Could you check a few things on this model? Use its own coordinates, in mm. A direction names the side the tool comes from. Give positions to 0.01 mm unless a question says otherwise; leave off trailing zeros. Order: outer loops, then holes, each group sorted by start corner. A loop starts at its lowest first (then second) coordinate and runs counter-clockwise, first axis right, second up.
from build123d import *

# Parameters (mm, degrees)
SKETCH_1_R          = 24
SKETCH_1_R_2        = 1.75
EXTRUDE_1_DEPTH     = 8
FILLET_1_R          = 10
FILLET_3_R          = 10
FILLET_8_R          = 23
FILLET_9_R          = 23
SKETCH_3_R          = 2
CUT_EXTRUDE_1_DEPTH = 196.43671136
RIB_1_REACH         = 197.437
SKETCH_6_WALL_W     = 465.474103638
SKETCH_6_WALL_H     = 8
EXTRUDE_START       = 8
SKETCH_11_W         = 116.312569084
SKETCH_11_H         = 40.000018321
SKETCH_11_R         = 2
EXTRUDE_2_DEPTH     = 8
FILLET_11_R         = 5


with BuildPart() as part:
    # 草图1 → 凸台-拉伸1 (new body)
    with BuildSketch(Plane.XY):
        with BuildLine():
            Line((-100, -20), (100, -20))
            ThreePointArc((100, -20), (189.532340636, 0), (100, 20))
            Line((100, 20), (-100, 20))
            Line((-100, 20), (-100, -20))
        make_face()
        with Locations((142.532340636, 0)):
            Circle(SKETCH_1_R, mode=Mode.SUBTRACT)
        with Locations((123.782340636, 32.475952642)):
            Circle(SKETCH_1_R_2, mode=Mode.SUBTRACT)
        with Locations((107.293867357, 12.825755375)):
            Circle(SKETCH_1_R_2, mode=Mode.SUBTRACT)
        with Locations((107.293867357, -12.825755375)):
            Circle(SKETCH_1_R_2, mode=Mode.SUBTRACT)
        with Locations((123.782340636, -32.475952642)):
            Circle(SKETCH_1_R_2, mode=Mode.SUBTRACT)
        with Locations((149.044147299, -36.930290738)):
            Circle(SKETCH_1_R_2, mode=Mode.SUBTRACT)
        with Locations((171.259007253, -24.104535363)):
            Circle(SKETCH_1_R_2, mode=Mode.SUBTRACT)
        with Locations((180.032340636, 0)):
            Circle(SKETCH_1_R_2, mode=Mode.SUBTRACT)
        with Locations((171.259007253, 24.104535363)):
            Circle(SKETCH_1_R_2, mode=Mode.SUBTRACT)
        with Locations((149.044147299, 36.930290738)):
            Circle(SKETCH_1_R_2, mode=Mode.SUBTRACT)
    extrude(amount=EXTRUDE_1_DEPTH)

    # 圆角1
    fillet_1_edges = [part.edges().sort_by_distance(p)[0] for p in [
        (-100, 20, 4),
    ]]
    fillet(fillet_1_edges, radius=FILLET_1_R)

    # 圆角3
    fillet_3_edges = [part.edges().sort_by_distance(p)[0] for p in [
        (-100, -20, 4),
    ]]
    fillet(fillet_3_edges, radius=FILLET_3_R)

    # 圆角8
    fillet_8_edges = [part.edges().sort_by_distance(p)[0] for p in [
        (100, -20, 4),
    ]]
    fillet(fillet_8_edges, radius=FILLET_8_R)

    # 圆角9
    fillet_9_edges = [part.edges().sort_by_distance(p)[0] for p in [
        (100, 20, 4),
    ]]
    fillet(fillet_9_edges, radius=FILLET_9_R)

    # 草图3 → 切除-拉伸1 (cut, through all)
    with BuildSketch(Plane.XY.offset(8)):
        with Locations((-86.637479545, 10)):
            Circle(SKETCH_3_R)
        with Locations((-86.610408267, -9.999981679)):
            Circle(SKETCH_3_R)
        with Locations((-76.637479545, 10)):
            Circle(SKETCH_3_R)
        with Locations((-76.610408267, -9.999981679)):
            Circle(SKETCH_3_R)
        with Locations((-46.637479545, 10)):
            Circle(SKETCH_3_R)
        with Locations((-46.610408267, -9.999981679)):
            Circle(SKETCH_3_R)
        with Locations((-36.637479545, 10)):
            Circle(SKETCH_3_R)
        with Locations((-36.610408267, -9.999981679)):
            Circle(SKETCH_3_R)
        with Locations((-6.637479545, 10)):
            Circle(SKETCH_3_R)
        with Locations((-6.610408267, -9.999981679)):
            Circle(SKETCH_3_R)
        with Locations((3.362520455, 10)):
            Circle(SKETCH_3_R)
        with Locations((3.389591733, -9.999981679)):
            Circle(SKETCH_3_R)
        with Locations((33.362520455, 10)):
            Circle(SKETCH_3_R)
        with Locations((33.389591733, -9.999981679)):
            Circle(SKETCH_3_R)
        with Locations((43.362520455, 10)):
            Circle(SKETCH_3_R)
        with Locations((43.389591733, -9.999981679)):
            Circle(SKETCH_3_R)
        with Locations((63.247313172, 10)):
            Circle(SKETCH_3_R)
        with Locations((84.747313172, 10)):
            Circle(SKETCH_3_R)
        with Locations((84.747313172, -11.5)):
            Circle(SKETCH_3_R)
        with Locations((63.247313172, -11.5)):
            Circle(SKETCH_3_R)
    extrude(amount=-CUT_EXTRUDE_1_DEPTH, mode=Mode.SUBTRACT)

    # 草图6 wall → 筋1 (add, up to next)
    with BuildSketch(Plane(origin=(69.41709698, 24.435714285, 8), x_dir=(0.992506131536, 0.122194839758, 0), z_dir=(-0.122194839758, 0.992506131536, 0)), mode=Mode.PRIVATE) as rib_1_sk1:
        with Locations((0, 4)):
            Rectangle(SKETCH_6_WALL_W, SKETCH_6_WALL_H)
    rib_1_tool1 = extrude(rib_1_sk1.sketch, amount=-RIB_1_REACH, mode=Mode.PRIVATE) - part.part
    add(rib_1_tool1.solids().sort_by_distance((69.41709698, 24.435714285, 8))[0])

    # 草图11 → 凸台-拉伸2 (add)
    with BuildSketch(Plane.XY.offset(8).offset(EXTRUDE_START)):
        with Locations((-1.623943906, 9.161e-06)):
            Rectangle(SKETCH_11_W, SKETCH_11_H)
        with Locations((-46.637479545, 10)):
            Circle(SKETCH_11_R, mode=Mode.SUBTRACT)
        with Locations((-36.637479545, 10)):
            Circle(SKETCH_11_R, mode=Mode.SUBTRACT)
        with Locations((-36.610408267, -9.999981679)):
            Circle(SKETCH_11_R, mode=Mode.SUBTRACT)
        with Locations((-46.610408267, -9.999981679)):
            Circle(SKETCH_11_R, mode=Mode.SUBTRACT)
        with Locations((-6.637479545, 10)):
            Circle(SKETCH_11_R, mode=Mode.SUBTRACT)
        with Locations((-6.610408267, -9.999981679)):
            Circle(SKETCH_11_R, mode=Mode.SUBTRACT)
        with Locations((3.389591733, -9.999981679)):
            Circle(SKETCH_11_R, mode=Mode.SUBTRACT)
        with Locations((3.362520455, 10)):
            Circle(SKETCH_11_R, mode=Mode.SUBTRACT)
        with Locations((33.362520455, 10)):
            Circle(SKETCH_11_R, mode=Mode.SUBTRACT)
        with Locations((43.362520455, 10)):
            Circle(SKETCH_11_R, mode=Mode.SUBTRACT)
        with Locations((43.389591733, -9.999981679)):
            Circle(SKETCH_11_R, mode=Mode.SUBTRACT)
        with Locations((33.389591733, -9.999981679)):
            Circle(SKETCH_11_R, mode=Mode.SUBTRACT)
    extrude(amount=-EXTRUDE_2_DEPTH)

    # 圆角11
    fillet_11_edges = [part.edges().sort_by_distance(p)[0] for p in [
        (56.532340636, 9.161e-06, 16),
        (-1.623943906, 20.000018321, 16),
        (-59.780228448, 9.161e-06, 16),
        (-1.623943906, -20, 16),
    ]]
    fillet(fillet_11_edges, radius=FILLET_11_R)


solid = part.part
Item 1: Imagine slicing it at C-C on z = 3. Give the number of separate pieces and of enclosed holes in the cut face, then the cut area to 3 significant figures.
Findings:
separate pieces: 1
enclosed holes: 30
area: 12,900 mm2
Item 2: Please list where these lines run through material, in increasing order: line 1 along Y through (x, z) = (-5.5, 3); line 2 along Z through (x, y) = (121.5, 23); line 3 along Y through (x, z) = (-29.5, 11.25).
Findings:
line 1: y = -20 to -11.66, -8.34 to 8.35, 11.65 to 20
line 2: z = 0 to 8
line 3: y = -19.99 to 19.99
Item 3: For faces 1 (the flat face through (-100, 0, 4)), 2 (the flat face through (-80, 0, 8)), 3 (the flat face through (-27, 20, 4)), which set-ups out of +Z, -Z, +X, -X, +Y, -Y let a thin tool reach every point of the face, with its end or its side?
Findings:
face 1: +Z, -Z, -X, +Y, -Y
face 2: +Z, -X, +Y, -Y
face 3: +Z, -Z, -X, +Y
Item 4: For pin 1 (20 mm diameter, centred on x = -89, y = -3, fed in from +Z); pin 2 (2.5 mm diameter, centred on x = 84.75, y = 10, fed in from -Z); pin 3 (1.5 mm diameter, centred on y = 1.5, z = 12.5, fed in from +X); pin 4 (1.5 mm diameter, centred on y = 2.5, z = 10, fed in from -X), each with a flat end and sliding along its axis, tell me the tip position at first contact or that it passes through.
Findings:
pin 1: stops at z = 8
pin 2: passes through
pin 3: stops at x = 56.48
pin 4: stops at x = -59.78
Item 5: Imagine slicing it at A-A on x = 140.5. List the corners of the cut face in (y, z) for me, then the cut area to 3 significant figures.
Findings:
outline: (-46.96, 0) - (-23.91, 0) - (-23.91, 8) - (-46.96, 8) - close; (23.91, 0) - (46.96, 0) - (46.96, 8) - (23.91, 8) - close
area: 369 mm2
Item 6: We'd pull the mould along X, two halves only. Please class faces 4 (the cylindrical face through (164.7, -9.2, 3.9)), 5 (the flat face through (-3, -20, 6)), 6 (the cylindrical face through (-58.35, 0.28, 14.5)), 7 (the cylindrical face through (189.504, -1.632, 3.944)): +X half, -X half, draft (parallel to the pull), parting line (faces both ways), or undercut.
Findings:
face 4: undercut
face 5: draft
face 6: -X half
face 7: parting line
